Autodesk Inventor part; units mm, degrees
ref_plane "YZ Plane" through (0, 0, 0) normal (1, 0, 0) x (0, 1, 0)
ref_plane "XZ Plane" through (0, 0, 0) normal (0, 1, 0) x (-1, 0, 0)
ref_plane "XY Plane" through (0, 0, 0) normal (0, 0, 1) x (1, 0, 0)
sketch "Sketch1" plane through (0, 0, 0) normal (0, 0, 1) x (1, 0, 0)
  circle A0 centre (0, 0) radius 20.32 construction
  circle A1 centre (0, 0) radius 22.86 construction
  circle A2 centre (24.5471, 44.4756) radius 30.48 construction
  circle A3 centre (-36.4129, 44.4756) radius 30.48 construction
  circle A4 centre (-36.4129, 44.4756) radius 33.02 construction
  line L0 (-15.4952, 18.9262) -> (-14.4815, 17.688)
  circle A5 centre (24.5471, 44.4756) radius 33.02 construction
  circle A6 centre (24.5471, 44.4756) radius 14.2875
  circle A7 centre (-36.4129, 44.4756) radius 14.2875
  circle A8 centre (0, 0) radius 14.2875
  circle A9 centre (24.5471, 44.4756) radius 19.1008 construction
  circle A10 centre (24.5471, 44.4756) radius 21.0058 construction
  circle A11 centre (-36.4129, 44.4756) radius 19.1008 construction
  circle A12 centre (-36.4129, 44.4756) radius 21.0058 construction
  line L1 (-36.4129, 44.4756) -> (-174.0993, 152.048) construction
  line L2 (24.5471, 44.4756) -> (162.2336, 152.048) construction
  circle A13 centre (-174.0993, 152.048) radius 14.2875
  circle A14 centre (162.2336, 152.048) radius 14.2875
  circle A15 centre (-174.0993, 152.048) radius 22.225 construction
  circle A16 centre (162.2336, 152.048) radius 22.225 construction
  line L3 (-160.4162, 169.5616) -> (-45.921, 80.1081)
  line L4 (-42.9811, 79.0958) -> (31.1154, 79.0958)
  arc A17 (31.1154, 79.0958) -> (34.0553, 80.1081) centre (31.1154, 83.871) ccw
  arc A18 (-45.921, 80.1081) -> (-42.9811, 79.0958) centre (-42.9811, 83.871) ccw
  line L5 (34.0553, 80.1081) -> (148.5505, 169.5616)
  line L6 (-36.4129, 79.0958) -> (-36.4129, 77.4956) construction
  arc A19 (177.8656, 136.2496) -> (148.5505, 169.5616) centre (162.2336, 152.048) ccw
  arc A20 (-160.4162, 169.5616) -> (-189.2001, 135.7411) centre (-174.0993, 152.048) ccw
  circle A21 centre (-105.2561, 98.2618) radius 2.0193
  circle A22 centre (0, -30.8102) radius 6.35 construction
  circle A23 centre (0, -30.8102) radius 2.0193
  line L7 (0, -22.86) -> (0, -24.4602)
  line L8 (-189.2001, 135.7411) -> (-4.3145, -35.4693)
  line L9 (177.8656, 136.2496) -> (4.4663, -35.324)
  arc A24 (-4.3145, -35.4693) -> (4.4663, -35.324) centre (0, -30.8102) ccw
  circle A25 centre (-105.2561, 98.2618) radius 6.35 construction
  circle A26 centre (93.3904, 98.2618) radius 6.35 construction
  circle A27 centre (93.3904, 98.2618) radius 2.0193
  circle A28 centre (-174.0993, 152.048) radius 50.8 construction
  circle A29 centre (162.2336, 152.048) radius 50.8 construction
  line L10 (-333.708, 192.5945) -> (-312.3217, 152.048) construction
  dimension "d0" = 40.64
  dimension "d3" = 2.54
  dimension "d9" = 60.96
  dimension "d10" = 2.54
  dimension "d12" = 1.6002
  dimension "d13" = 28.575
  dimension "d14" = 38.2016
  dimension "d15" = 42.0116
  dimension "d16" = 174.7266
  dimension "d17" = 104
  dimension "d18" = 28.575
  dimension "d24" = 44.45
  dimension "d25" = 44.45
  dimension "d37" = 4.7752
  dimension "d38" = 1.6002
  dimension "d39" = 4.0386
  dimension "d40" = 12.7
  dimension "d41" = 4.0386
  dimension "d42" = 1.6002
  dimension "d43" = 12.7
  dimension "d44" = 12.7
  dimension "d45" = 4.0386
  dimension "d46" = 87.3633
  dimension "d47" = 87.3633
  dimension "d48" = 101.6
  dimension "d49" = 101.6
extrude "Extrusion1" add sketch "Sketch1" along normal mid plane 6.35
properties part number "Gearbox #2 Plate" material "Aluminum 6061"
Geometry check sheet. Reference: the model listing, model coordinates, mm. A direction names the side the tool comes from. Give positions to 0.01 mm unless a question says otherwise; leave off trailing zeros. Order: outer loops, then holes, each group sorted by start corner. A loop starts at its lowest first (then second) coordinate and runs counter-clockwise, first axis right, second up. Notation, with made-up numbers: (81.25, 36) -> (98.25, 36) arc R8 cw to (98.25, 48) -> close; hole circle Ø2 at (1, -15). An arc over 180 degrees is marked (long way). Write each question's results on one line, items separated by ' | '. Start each with the question number.
(1) Gauge pin test, flat ends, axial feed: P1, Ø2, axis at y = 102, z = 0, coming from the +X side; P2, Ø3, axis at y = 9.5, z = 0.5, coming from the +X side; P3, Ø1.5, axis at x = 89, z = -1, coming from the -Y side. Record the tip position at first contact, or that the pin passes through.
(2) Sectioned sample at D-D (x = 71). Enter the section's corners in (y, z) (3 decimals), plus the area to 3 significant figures.
(3) Sectioned sample at A-A (y = 86.5). Enter the section's corners in (x, z) (3 decimals), plus the area to 3 significant figures.
(4) Scan lines: line 1 (Y direction, x = 0, z = 0.75); line 2 (X direction, y = 143.5, z = 1.5); line 3 (X direction, y = 142, z = -0.75). Record each from-to range of solid material in increasing order.
(5) Mould release check, pull along X, two halves, no side actions. Record for faces 3 (the face through (92.38, 51.664, -0.044)), 4 (the face through (-98.051, 51.334, -0.044)), 5 (the face through (-7, 77, 3.175)), 6 (the face through (178.603, 167.081, -0.044)): pulls with the +X half, pulls with the -X half, needs draft (parallel to the pull), parting line crosses it, or undercut.
(6) Sectioned sample at B-B (z = -0.75). Give the number of separate pieces and of enclosed holes in the cut face, plus the area to 3 significant figures.
(7) Sectioned sample at C-C (y = 114). Enter the section's corners in (x, z) (3 decimals), plus the area to 3 significant figures.
(8) Access from +Z, -Z, +X, -X, +Y, -Y to the whole of each face (thin tool, end or side, straight path). Record for faces 1 (the face through (-14.274, -0.628, -0.044)), 2 (the face through (90.5, 124.21, -0.04)).
Answer below:
1) P1: x = 144.26 | P2: x = 51.28 | P3: y = 47.58
2) outline: (30.509, -3.175) -> (108.972, -3.175) -> (108.972, 3.175) -> (30.509, 3.175) -> close | area: 498 mm2
3) outline: (-136.026, -3.175) -> (-54.102, -3.175) -> (-54.102, 3.175) -> (-136.026, 3.175) -> close; (42.237, -3.175) -> (127.587, -3.175) -> (127.587, 3.175) -> (42.237, 3.175) -> close | area: 1,060 mm2
4) line 1: -37.16 to -32.83, -28.79 to -14.29, 14.29 to 79.1 | line 2: -194.61 to -185.55, -162.65 to -127.06, 115.19 to 150.79, 173.68 to 182.75 | line 3: -193.92 to -184.26, -163.94 to -125.14, 113.27 to 152.08, 172.39 to 182.06
5) face 3: pulls with the +X half | face 4: pulls with the -X half | face 5: needs draft | face 6: undercut
6) separate pieces: 1 | enclosed holes: 8 | area: 24,300 mm2
7) outline: (-165.722, -3.175) -> (-89.301, -3.175) -> (-89.301, 3.175) -> (-165.722, 3.175) -> close; (77.435, -3.175) -> (155.379, -3.175) -> (155.379, 3.175) -> (77.435, 3.175) -> close | area: 980 mm2
8) face 1: +Z, -Z | face 2: +Z, -Z, +Y
